Could you check a few things on this model? Use its own coordinates, in mm. Round coordinates to 2 decimals unless told otherwise and drop trailing zeros. Loops run counter-clockwise (first coordinate to the right, second up) from the corner with the lowest first, then second, coordinate; pieces in that order, holes last. Notation, with made-up numbers: (-0.5, 65) -> (43.5, 65) arc R19 cw to (43.5, 77) -> close; hole circle Ø11 at (27, 60). An arc over 180 degrees is marked (long way). One line per item, written item: value.
from build123d import *

# Parameters (mm, degrees)
PAD004_DEPTH    = 30
SKETCH018_R     = 2.5
POCKET007_DEPTH = 100.001
SKETCH019_R     = 30
POCKET008_DEPTH = 100.001
PAD005_DEPTH    = 90


with BuildPart() as part:
    # Sketch016 → Pad004 (new body)
    with BuildSketch(Plane.XY):
        Polygon((10, -50), (-10, -50), (-10, 50), (90, 50), (90, 40), (10, 40), align=None)
    extrude(amount=PAD004_DEPTH)

    # Sketch018 → Pocket007 (cut, through all)
    with BuildSketch(Plane(origin=(0, 50, 0), x_dir=(-1, 0, 0), z_dir=(0, 1, 0))):
        with Locations((-80, 15)):
            Circle(SKETCH018_R)
    extrude(amount=-POCKET007_DEPTH, mode=Mode.SUBTRACT)

    # Sketch019 (on Face1 of Pocket007) → Pocket008 (cut, through all)
    with BuildSketch(Plane.XZ.offset(50)):
        with Locations((-35.69, 15)):
            Circle(SKETCH019_R)
    extrude(amount=-POCKET008_DEPTH, mode=Mode.SUBTRACT)

    # Sketch020 (on Face7 of Pocket008) → Pad005 (join)
    with BuildSketch(Plane.XZ.offset(-40)):
        with BuildLine():
            Line((10, 0), (10, 30))
            ThreePointArc((10, 0), (14.019238, 15), (10, 30))
        make_face()
    extrude(amount=PAD005_DEPTH)


with BuildPart() as part_1:
    # Body005 placement: moved
    add(part.part.moved(Location((-69, 36, -15))))


solid = part_1.part
(1) If I drill on L1, parallel to Z at x = 11, y = 79; L2, parallel to Y at x = -9, z = -10; L3, parallel to X at y = 19.5, z = 1, over which ranges is the centre line in solid material (lowest first)?
Recorded:
L1: -15 to -2.5, 2.5 to 15
L2: 76 to 86
L3: -74.71 to -55
(2) I'm going to push flat-ended pins straight in: pin 1 Ø10 at (y, z) = (66, 10.5) entering from +X; pin 2 Ø5 at (y, z) = (17.5, 8.5) entering from -X; pin 3 Ø5 at (x, z) = (-40.5, -12) entering from -Y. Where does each tip first touch, or does it pass through?
Recorded:
pin 1: x = -55.49
pin 2: x = -76.78
pin 3: y = 76
(3) If we section it at D-D, the plane y = 64.5: Please give me the cut outline in (x, z), then the cut area to 3 significant figures.
Recorded:
outline: (-78.71, -15) -> (-59, -15) arc R30 ccw to (-59, 15) -> (-78.71, 15) arc R30 cw to start
area: 591 mm²
(4) If we section it at B-B, the plane z = 0: Please give me the cut outline in (x, y), then the cut area to 3 significant figures.
Recorded:
outline: (-74.69, -14) -> (-54.98, -14) -> (-54.98, 76) -> (8.5, 76) -> (8.5, 86) -> (-74.69, 86) -> close; (13.5, 76) -> (21, 76) -> (21, 86) -> (13.5, 86) -> close
area: 2,680 mm²
(5) If we section it at A-A, the plane x = 11: Please give me the cut outline in (y, z).
Recorded:
outline: (76, -15) -> (86, -15) -> (86, -2.5) -> (76, -2.5) -> close; (76, 2.5) -> (86, 2.5) -> (86, 15) -> (76, 15) -> close
(6) If we section it at C-C, the plane x = -53.5: Please give me the cut outline in (y, z), then the cut area to 3 significant figures.
Recorded:
outline: (76, -15) -> (86, -15) -> (86, 15) -> (76, 15) -> close
area: 300 mm²
(7) Thinking about a two-plate mould opening in X: for faces 1 (the face through (-18, 76, 0)), 2 (the face through (13, 81.1, -1.5)), 3 (the face through (-54.98, 31.63, -0.22)), which applies, released by +X, released by -X, zero draft, split by the parting line, or undercut?
Recorded:
face 1: zero draft
face 2: undercut
face 3: released by +X
